CAD build for the part. Positions are in the model's coordinates, mm. Face numbers are marked on the shaded views. A direction names the side the tool comes from. Round coordinates to 2 decimals unless told otherwise and drop trailing zeros. Order: outer loops, then holes, each group sorted by start corner. A loop starts at its lowest first (then second) coordinate and runs counter-clockwise, first axis right, second up. Notation, with made-up numbers: M 46,82 L 66,82 A24 cw 66,102 Z; hole C -37,79 d11. An arc over 180 degrees is marked long. Answer as a JSON object with one key per item and string values.
```python
from build123d import *

# Parameters (mm, degrees)
BOSS_EXTRUDE1_DEPTH      = 2.6
BOSS_EXTRUDE2_DEPTH      = 4
SKETCH3_W                = 3
SKETCH3_H                = 5.2
BOSS_EXTRUDE3_DEPTH      = 8
BOSS_EXTRUDE4_DEPTH      = 2.6
CHAMFER1_SIZE            = 1
MIRROR2_COPY_1_DEPTH     = 4
CHAMFER1_OF_MIRROR2_SIZE = 1
CHAMFER2_SIZE            = 1


with BuildPart() as part:
    # Sketch1 → Boss-Extrude1 (new, symmetric)
    with BuildSketch(Plane(origin=(0, 0, 0), x_dir=(1, 0, 0), z_dir=(0, 1, 0))):
        Polygon((0, 0), (-2.828427125, -2.828427125), (-1.414213562, -4.242640687), (-7.071067812, -9.899494937), (-8.485281374, -8.485281374), (-11.313708499, -11.313708499), (-8.485281374, -14.142135624), (-5.656854249, -11.313708499), (5.656854249, -11.313708499), (8.485281374, -14.142135624), (11.313708499, -11.313708499), (8.485281374, -8.485281374), (7.071067812, -9.899494937), (1.414213562, -4.242640687), (2.828427125, -2.828427125), align=None)
    extrude(amount=BOSS_EXTRUDE1_DEPTH, both=True)

    # Sketch2 → Boss-Extrude2 (add)
    with BuildSketch(Plane(origin=(-11.313708499, 0, 11.313708499), x_dir=(0.7071067811865501, 0, 0.7071067811865449), z_dir=(-0.7071067811865449, 0, 0.7071067811865501))):
        Polygon((-1.5, -1.25), (-1.5, -2.6), (-4.5, -2.6), (-4.5, 2.6), (-1.5, 2.6), (-1.5, 1.25), (0, 1.25), (0, -1.25), align=None)
    boss_extrude2 = extrude(amount=-BOSS_EXTRUDE2_DEPTH)

    # Mirror1: Boss-Extrude2 across plane
    add(boss_extrude2.mirror(Plane(origin=(-5.656854249, 0, 5.656854249), x_dir=(0.707106781186549, 0, 0.707106781186546), z_dir=(-0.707106781186546, 0, 0.707106781186549))))

    # Sketch3 → Boss-Extrude3 (add)
    with BuildSketch(Plane(origin=(-2.828427125, 0, 2.828427125), x_dir=(0.7071067811865493, 0, 0.7071067811865457), z_dir=(-0.7071067811865457, 0, 0.7071067811865493))):
        with Locations((-3, 0)):
            Rectangle(SKETCH3_W, SKETCH3_H)
    boss_extrude3 = extrude(amount=BOSS_EXTRUDE3_DEPTH)

    # Sketch4 → Boss-Extrude4 (add, symmetric)
    with BuildSketch(Plane(origin=(0, 0, 0), x_dir=(1, 0, 0), z_dir=(0, 1, 0))):
        with BuildLine():
            Line((-7.778174593, -9.192388155), (-7.071067812, -9.899494937))
            Line((-7.071067812, -9.899494937), (-6.69213043, -9.520557555))
            ThreePointArc((-6.69213043, -9.520557555), (-6.068382545, -6.139500295), (-3.050994148, -4.491478184))
            ThreePointArc((-3.050994148, -4.491478184), (-2.579589628, -3.964431908), (-3.106635904, -3.493027387))
            ThreePointArc((-3.106635904, -3.493027387), (-6.695410435, -5.315669399), (-7.778174593, -9.192388155))
        make_face()
    boss_extrude4 = extrude(amount=BOSS_EXTRUDE4_DEPTH, both=True)

    # Chamfer1
    chamfer1_edges = [part.edges().sort_by_distance(p)[0] for p in [
        (-8.838834765, -2.6, 2.474873734),
        (-8.838834765, 2.6, 2.474873734),
        (-14.495689014, 0, 8.131727984),
        (-13.435028843, -2.6, 9.192388155),
        (-13.435028843, 2.6, 9.192388155),
        (-3.181980515, 0, -3.181980515),
        (-2.121320344, -2.6, -2.121320344),
        (-2.121320344, 2.6, -2.121320344),
    ]]
    chamfer(chamfer1_edges, length=CHAMFER1_SIZE)

    # Mirror2: Boss-Extrude2, Boss-Extrude3, Boss-Extrude4 across plane
    add(boss_extrude2.mirror(Plane(origin=(0, 0, 0), x_dir=(0, 0, 1), z_dir=(1, 0, 0))))
    add(boss_extrude3.mirror(Plane(origin=(0, 0, 0), x_dir=(0, 0, 1), z_dir=(1, 0, 0))))
    add(boss_extrude4.mirror(Plane(origin=(0, 0, 0), x_dir=(0, 0, 1), z_dir=(1, 0, 0))))

    # Mirror2 copy 1 sketch → Mirror2 copy 1 (add)
    with BuildSketch(Plane(origin=(0, 0, 0), x_dir=(-0.7071067811865479, 0, 0.7071067811865471), z_dir=(-0.7071067811865471, 0, -0.7071067811865479))):
        Polygon((-1.5, -1.25), (-1.5, -2.6), (-4.5, -2.6), (-4.5, 2.6), (-1.5, 2.6), (-1.5, 1.25), (0, 1.25), (0, -1.25), align=None)
    extrude(amount=-MIRROR2_COPY_1_DEPTH)

    # Chamfer1 of Mirror2
    chamfer1_of_mirror2_edges = [part.edges().sort_by_distance(p)[0] for p in [
        (8.838834765, -2.6, 2.474873734),
        (8.838834765, 2.6, 2.474873734),
        (14.495689014, 0, 8.131727984),
        (13.435028843, -2.6, 9.192388155),
        (13.435028843, 2.6, 9.192388155),
        (3.181980515, 0, -3.181980515),
        (2.121320344, -2.6, -2.121320344),
        (2.121320344, 2.6, -2.121320344),
    ]]
    chamfer(chamfer1_of_mirror2_edges, length=CHAMFER1_OF_MIRROR2_SIZE)

    # Chamfer2
    # the kernel refuses this chamfer: 1 mm, written as the material it takes off along each edge
    with BuildSketch(Plane(origin=(11.313708499, -5.171682988, 11.313708499), x_dir=(-0.6873969152646685, 0, 0.7262819568766788), z_dir=(0, 1, 0)), Plane(origin=(11.313708499, 1.25, 11.313708499), x_dir=(-0.6873969152646685, 0, 0.7262819568766788), z_dir=(0, 1, 0)), Plane(origin=(0, 5.171682988, 0), x_dir=(-0.7262819568766743, 0, 0.6873969152646733), z_dir=(0, -1, 0)), Plane(origin=(-11.313708499, -5.171682988, 11.313708499), x_dir=(0.6873969152646597, 0, -0.7262819568766873), z_dir=(0, 1, 0)), Plane(origin=(0, -1.25, 0), x_dir=(-0.7262819568766743, 0, 0.6873969152646733), z_dir=(0, -1, 0))) as chamfer2_piece_1:
        Polygon((CHAMFER2_SIZE * 0.999621916911, -CHAMFER2_SIZE * 0.0274958766106), (-CHAMFER2_SIZE * 0.0274958766106, -CHAMFER2_SIZE * 0.999621916911), (0, 0), align=None)
    extrude(amount=3.921682988, mode=Mode.SUBTRACT)
    with BuildSketch(Plane(origin=(11.313708499, -5.171682988, 11.313708499), x_dir=(-0.6873969152646685, 0, 0.7262819568766788), z_dir=(0, 1, 0))) as chamfer2_piece_2_section:
        Polygon((CHAMFER2_SIZE * 0.999621916911, -CHAMFER2_SIZE * 0.0274958766106), (-CHAMFER2_SIZE * 0.0274958766106, -CHAMFER2_SIZE * 0.999621916911), (0, 0), align=None)
    chamfer2_piece_2 = extrude(amount=6.493365976, mode=Mode.PRIVATE)
    chamfer2_piece_2 = split(chamfer2_piece_2, bisect_by=Plane(origin=(10.847309879, 1.25, 11.313708499), z_dir=(0, 1, 0)), keep=Keep.TOP, mode=Mode.PRIVATE)
    add(chamfer2_piece_2, mode=Mode.SUBTRACT)
    with BuildSketch(Plane(origin=(11.313708499, -1.321682988, 11.313708499), x_dir=(-0.6873969152646685, 0, 0.7262819568766788), z_dir=(0, 1, 0))) as chamfer2_piece_3_section:
        Polygon((CHAMFER2_SIZE * 0.999621916911, -CHAMFER2_SIZE * 0.0274958766106), (-CHAMFER2_SIZE * 0.0274958766106, -CHAMFER2_SIZE * 0.999621916911), (0, 0), align=None)
    chamfer2_piece_3 = extrude(amount=6.493365976, mode=Mode.PRIVATE)
    chamfer2_piece_3 = split(chamfer2_piece_3, bisect_by=Plane(origin=(10.847309879, -1.25, 11.313708499), z_dir=(0, -1, 0)), keep=Keep.TOP, mode=Mode.PRIVATE)
    add(chamfer2_piece_3, mode=Mode.SUBTRACT)
    with BuildSketch(Plane(origin=(8.485281374, -5.171682988, 14.142135624), x_dir=(0.7262819568766956, 0, -0.6873969152646507), z_dir=(0, 1, 0))) as chamfer2_piece_4:
        Polygon((CHAMFER2_SIZE * 0.999621916911, CHAMFER2_SIZE * 0.0274958766106), (-CHAMFER2_SIZE * 0.0274958766106, CHAMFER2_SIZE * 0.999621916911), (0, 0), align=None)
    extrude(amount=10.343365976, mode=Mode.SUBTRACT)
    with BuildSketch(Plane(origin=(-8.485281374, -5.171682988, 14.142135624), x_dir=(-0.7262819568766898, 0, -0.687396915264657), z_dir=(0, 1, 0))) as chamfer2_piece_5:
        Polygon((CHAMFER2_SIZE * 0.999621916911, -CHAMFER2_SIZE * 0.0274958766106), (-CHAMFER2_SIZE * 0.0274958766106, -CHAMFER2_SIZE * 0.999621916911), (0, 0), align=None)
    extrude(amount=10.343365976, mode=Mode.SUBTRACT)
    with BuildSketch(Plane(origin=(-11.313708499, -1.321682988, 11.313708499), x_dir=(0.6873969152646623, 0, 0.7262819568766848), z_dir=(0, 1, 0))) as chamfer2_piece_6_section:
        Polygon((CHAMFER2_SIZE * 0.999621916911, CHAMFER2_SIZE * 0.0274958766106), (-CHAMFER2_SIZE * 0.0274958766106, CHAMFER2_SIZE * 0.999621916911), (0, 0), align=None)
    chamfer2_piece_6 = extrude(amount=6.493365976, mode=Mode.PRIVATE)
    chamfer2_piece_6 = split(chamfer2_piece_6, bisect_by=Plane(origin=(-10.847309879, -1.25, 11.313708499), z_dir=(0, -1, 0)), keep=Keep.TOP, mode=Mode.PRIVATE)
    add(chamfer2_piece_6, mode=Mode.SUBTRACT)
    with BuildSketch(Plane(origin=(-11.313708499, 1.25, 11.313708499), x_dir=(0.6873969152646623, 0, 0.7262819568766848), z_dir=(0, 1, 0))) as chamfer2_piece_7:
        Polygon((CHAMFER2_SIZE * 0.999621916911, CHAMFER2_SIZE * 0.0274958766106), (-CHAMFER2_SIZE * 0.0274958766106, CHAMFER2_SIZE * 0.999621916911), (0, 0), align=None)
    extrude(amount=3.921682988, mode=Mode.SUBTRACT)
    with BuildSketch(Plane(origin=(0, 5.171682988, 0), x_dir=(-0.7262819568766743, 0, 0.6873969152646733), z_dir=(0, -1, 0))) as chamfer2_piece_8_section:
        Polygon((CHAMFER2_SIZE * 0.999621916911, -CHAMFER2_SIZE * 0.0274958766106), (-CHAMFER2_SIZE * 0.0274958766106, -CHAMFER2_SIZE * 0.999621916911), (0, 0), align=None)
    chamfer2_piece_8 = extrude(amount=6.493365976, mode=Mode.PRIVATE)
    chamfer2_piece_8 = split(chamfer2_piece_8, bisect_by=Plane(origin=(0, -1.25, 0.46639862), z_dir=(0, -1, 0)), keep=Keep.TOP, mode=Mode.PRIVATE)
    add(chamfer2_piece_8, mode=Mode.SUBTRACT)
    with BuildSketch(Plane(origin=(-11.313708499, -5.171682988, 11.313708499), x_dir=(0.6873969152646597, 0, -0.7262819568766873), z_dir=(0, 1, 0))) as chamfer2_piece_9_section:
        Polygon((CHAMFER2_SIZE * 0.999621916911, -CHAMFER2_SIZE * 0.0274958766106), (-CHAMFER2_SIZE * 0.0274958766106, -CHAMFER2_SIZE * 0.999621916911), (0, 0), align=None)
    chamfer2_piece_9 = extrude(amount=6.493365976, mode=Mode.PRIVATE)
    chamfer2_piece_9 = split(chamfer2_piece_9, bisect_by=Plane(origin=(-10.847309879, 1.25, 11.313708499), z_dir=(0, 1, 0)), keep=Keep.TOP, mode=Mode.PRIVATE)
    add(chamfer2_piece_9, mode=Mode.SUBTRACT)
    with BuildSketch(Plane(origin=(0, 1.321682988, 0), x_dir=(-0.7262819568766743, 0, 0.6873969152646733), z_dir=(0, -1, 0))) as chamfer2_piece_10_section:
        Polygon((CHAMFER2_SIZE * 0.999621916911, -CHAMFER2_SIZE * 0.0274958766106), (-CHAMFER2_SIZE * 0.0274958766106, -CHAMFER2_SIZE * 0.999621916911), (0, 0), align=None)
    chamfer2_piece_10 = extrude(amount=6.493365976, mode=Mode.PRIVATE)
    chamfer2_piece_10 = split(chamfer2_piece_10, bisect_by=Plane(origin=(0, 1.25, 0.46639862), z_dir=(0, 1, 0)), keep=Keep.TOP, mode=Mode.PRIVATE)
    add(chamfer2_piece_10, mode=Mode.SUBTRACT)


solid = part.part
```
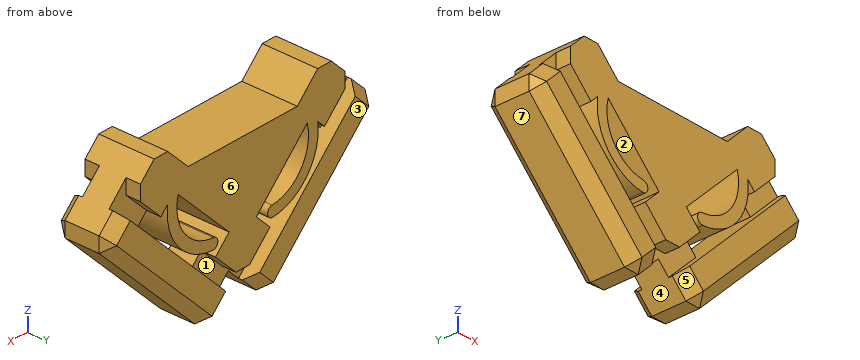
Item 1: Saw through at D-D on z = 1.5. List the corners of the cut face in (x, y), and give its area (3 significant figures).
Worked answers:
{"outline": "M -7.86,-1.6 L -6.45,-2.6 L -3.62,-2.6 L -3.62,-1.25 L -1.5,-1.25 L -1.5,-2.6 L 1.5,-2.6 L 1.5,-1.25 L 3.62,-1.25 L 3.62,-2.6 L 6.45,-2.6 L 7.86,-1.6 L 7.86,1.6 L 6.45,2.6 L 3.62,2.6 L 3.62,1.25 L 1.5,1.25 L 1.5,2.6 L -1.5,2.6 L -1.5,1.25 L -3.62,1.25 L -3.62,2.6 L -6.45,2.6 L -7.86,1.6 Z", "area": "67.5 mm2"}
Item 2: Saw through at C-C on z = 5.5. List the corners of the cut face in (x, y), and give its area (3 significant figures).
Worked answers:
{"outline": "M -11.86,-1.6 L -10.45,-2.6 L -7.62,-2.6 L -7.62,2.6 L -10.45,2.6 L -11.86,1.6 Z; M -6.84,-2.6 L -5.49,-2.6 L -5.49,2.6 L -6.84,2.6 Z; M -2.67,-2.6 L 2.67,-2.6 L 2.67,2.6 L -2.67,2.6 Z; M 5.49,-2.6 L 6.84,-2.6 L 6.84,2.6 L 5.49,2.6 Z; M 7.62,-2.6 L 10.45,-2.6 L 11.86,-1.6 L 11.86,1.6 L 10.45,2.6 L 7.62,2.6 Z", "area": "83.1 mm2"}
Item 3: Wall check: line 1 along X through (y, z) = (-0.15, 2.25); line 2 along X through (y, z) = (-1.1, 4); line 3 along X through (y, z) = (-0.6, 6). Give the ranges that are in metal, low to high. Write a range as [from, to].
Worked answers:
{"line 1": "x = [-8.61, -4.37], [-3.41, 3.41], [4.37, 8.61]", "line 2": "x = [-10.36, -6.12], [-5.04, -2.58], [-1.66, 1.66], [2.58, 5.04], [6.12, 10.36]", "line 3": "x = [-12.36, -8.12], [-7.17, -5.96], [-3.17, 3.17], [5.96, 7.17], [8.12, 12.36]"}
Item 4: 3-axis set-ups, long thin cutter, end or side, ignore diameter. For the marked faces 1, 2, 3 and 4: which of +Z, -Z, +X, -X, +Y, -Y reach the whole face in a straight line?
Worked answers:
{"face 1": "+Y", "face 2": "+Y, -Y", "face 3": "+Z, -Z, +X, -X, +Y", "face 4": "-Z, +Y, -Y"}
Item 5: Saw through at A-A on y = -0.85. State how many separate pieces and enclosed holes the cut face has, and give its area (3 significant figures).
Worked answers:
{"separate pieces": "1", "enclosed holes": "2", "area": "246 mm2"}
Item 6: Two-plate mould, pull along X, no slides. Class the marked faces 5, 6 and 7: released by +X, released by -X, zero draft, split by the parting line, or undercut.
Worked answers:
{"face 5": "undercut", "face 6": "zero draft", "face 7": "released by -X"}
Item 7: Drop flat-ended pins along their axis: pin 1 Ø0.7 at (y, z) = (1.5, 11.5) entering from -X; pin 2 Ø0.7 at (y, z) = (2, 11) entering from +X; pin 3 Ø1 at (x, z) = (0, -0.5) entering from -Y. Give the stop position or say it passes through.
Worked answers:
{"pin 1": "stops at x = -11.37", "pin 2": "stops at x = 10.61", "pin 3": "stops at y = -1.25"}
Item 8: Saw through at B-B on x = -5.25. List the corners of the cut face in (y, z).
Worked answers:
{"outline": "M -2.6,0.3 L -1.6,-1.11 L 1.6,-1.11 L 2.6,0.3 L 2.6,3.13 L -2.6,3.13 Z; M -2.6,4.11 L 2.6,4.11 L 2.6,5.3 L -2.6,5.3 Z; M -2.6,8.08 L 2.6,8.08 L 2.6,11.31 L -2.6,11.31 Z"}
